from build123d import *

# Parameters (mm, degrees)
SKETCH1_R           = 1.27
BOSS_EXTRUDE2_DEPTH = 3.175


with BuildPart() as part:
    # Sketch1 → Boss-Extrude2 (new body)
    with BuildSketch(Plane(origin=(0, 0, 0), x_dir=(1, 0, 0), z_dir=(0, 1, 0))):
        with BuildLine():
            ThreePointArc((-175.915621646, 29.519008442), (-181.461271413, 31.81826883), (-183.753097882, 37.366994908))
            Line((-183.753097882, 37.366994908), (-183.753097882, 134.805535228))
            ThreePointArc((-183.753097882, 134.805535228), (-181.458407426, 140.352437247), (-175.91562747, 142.657066645))
            Line((-175.91562747, 142.657066645), (-117.135020463, 142.660762281))
            ThreePointArc((-117.135020463, 142.660762281), (-111.588130828, 140.360246871), (-109.29759004, 134.809230866))
            Line((-109.29759004, 134.809230866), (-109.29759004, 37.37053719))
            ThreePointArc((-109.29759004, 37.37053719), (-111.597249567, 31.81866797), (-117.149118786, 29.519008442))
            Line((-117.149118786, 29.519008442), (-175.915621646, 29.519008442))
        make_face()
        with Locations(Location((-126.972959073, 129.95775743, 0), (0, 0, 270))):
            Circle(SKETCH1_R, mode=Mode.SUBTRACT)
        with Locations(Location((-164.472977249, 128.29201107, 0), (0, 0, 270))):
            Circle(SKETCH1_R, mode=Mode.SUBTRACT)
        with Locations(Location((-166.159897821, 90.761182378, 0), (0, 0, 270))):
            Circle(SKETCH1_R, mode=Mode.SUBTRACT)
        with Locations(Location((-126.972959075, 90.761489089, 0), (0, 0, 270))):
            Circle(SKETCH1_R, mode=Mode.SUBTRACT)
        with Locations(Location((-116.329373394, 75.456747577, 0), (0, 0, 270))):
            Circle(SKETCH1_R, mode=Mode.SUBTRACT)
        with Locations(Location((-121.602318573, 63.673415864, 0), (0, 0, 270))):
            Circle(SKETCH1_R, mode=Mode.SUBTRACT)
        with Locations(Location((-161.416515799, 75.608057078, 0), (0, 0, 270))):
            Circle(SKETCH1_R, mode=Mode.SUBTRACT)
        with Locations(Location((-177.85310358, 75.456747579, 0), (0, 0, 270))):
            Circle(SKETCH1_R, mode=Mode.SUBTRACT)
        with Locations(Location((-174.718127663, 47.58354115, 0), (0, 0, 270))):
            Circle(SKETCH1_R, mode=Mode.SUBTRACT)
        with Locations(Location((-122.379809257, 47.976111584, 0), (0, 0, 270))):
            Circle(SKETCH1_R, mode=Mode.SUBTRACT)
        with Locations(Location((-121.602318574, 41.767430359, 0), (0, 0, 270))):
            Circle(SKETCH1_R, mode=Mode.SUBTRACT)
        with Locations(Location((-162.435290361, 37.763153633, 0), (0, 0, 270))):
            Circle(SKETCH1_R, mode=Mode.SUBTRACT)
        with BuildLine():
            ThreePointArc((-144.679570761, 140.490425994), (-146.605093484, 141.290423511), (-148.531606371, 140.492813408))
            Line((-148.531606371, 140.492813408), (-176.798615575, 112.209681509))
            ThreePointArc((-176.798615575, 112.209681509), (-177.56091066, 110.280604208), (-176.801172002, 108.350518665))
            Line((-176.801172002, 108.350518665), (-148.569167296, 80.0322861))
            ThreePointArc((-148.569167296, 80.0322861), (-146.643487849, 79.232224846), (-144.71682032, 80.029903714))
            Line((-144.71682032, 80.029903714), (-116.449969407, 108.313038257))
            ThreePointArc((-116.449969407, 108.313038257), (-115.650538135, 110.242134618), (-116.447583058, 112.172218171))
            Line((-116.447583058, 112.172218171), (-144.679570761, 140.490425994))
        make_face(mode=Mode.SUBTRACT)
    extrude(amount=BOSS_EXTRUDE2_DEPTH)


solid = part.part
The listing builds one solid part. Answer for the finished solid, in the listing's coordinates (mm). A direction names the side the tool comes from. Coordinates: 2 decimals unless noted, no trailing zeros. Write each loop counter-clockwise with the first axis right and the second up, starting at its lowest first coordinate (ties: lowest second). Pieces come first, ordered by that corner, then holes. Notation, with made-up numbers: M -4.75,54.5 L 8.25,54.5 A7 cw 8.25,67.5 Z; hole C -36.75,45.5 d1. An arc over 180 degrees is marked long. Use one line per item in the form item = value.
Item 1: Find section B-B, the plane x = -147. Give the vertices of the cut face in (y, z) (3 decimals), plus the area to 3 significant figures.
Model answer:
outline = M 0,-142.659 L 3.175,-142.659 L 3.175,-141.262 L 0,-141.262 Z; M 0,-79.256 L 3.175,-79.256 L 3.175,-29.519 L 0,-29.519 Z
area = 162 mm2
Item 2: Find section C-C, the plane y = 1.95. Give the number of separate pieces and of enclosed holes in the cut face, plus the area to 3 significant figures.
Model answer:
separate_pieces = 1
enclosed_holes = 13
area = 6,250 mm2
Item 3: The mould has two halves that part along X. Classify faces 3 (the face through (-146, 0, -74)), 4 (the face through (-163.675, 1.565, -38.038)), 5 (the face through (-111.65, 1.57, -140.42)), 6 (the face through (-165.78, 1.57, -89.55)): released by +X, released by -X, zero draft, split by the parting line, or undercut.
Model answer:
face_3 = zero draft
face_4 = undercut
face_5 = released by +X
face_6 = undercut
Item 4: For faces 1 (the face through (-181.52, 1.57, -140.29)), 2 (the face through (-130.781, 1.565, -93.973)), determine the directions among +Z, -Z, +X, -X, +Y, -Y from which every point of the face is accessible in a straight line to the end or side of a thin tool.
Model answer:
face_1 = -Z, -X, +Y, -Y
face_2 = +Y, -Y
Item 5: Given P1, Ø1, axis at x = -170, y = 2.5, coming from the -Z side, flat-ended and moving along its own axis, determine where the tip first touches the part or whether it passes through.
Model answer:
P1 = -142.66
Item 6: Find section A-A, the plane z = -113.5. Give the vertices of the cut face in (x, y) (3 decimals).
Model answer:
outline = M -183.753,0 L -175.509,0 L -175.509,3.175 L -183.753,3.175 Z; M -117.771,0 L -109.298,0 L -109.298,3.175 L -117.771,3.175 Z
Item 7: Find the intervals of material crossed by probe 1 along X at (y, z) = (1.45, -110.5); probe 2 along X at (y, z) = (1, -76.5); probe 3 along Z at (x, y) = (-122.5, 1.6), in increasing order.
Model answer:
probe_1 = -183.75 to -177.55, -115.66 to -109.3
probe_2 = -183.75 to -178.58, -177.13 to -162.32, -160.51 to -117.05, -115.61 to -109.3
probe_3 = -142.66 to -118.24, -102.26 to -64.57, -62.78 to -49.24, -46.71 to -42.67, -40.87 to -29.52
